Input: part model. Units: mm. Frame: model coordinates. Face numbers are marked on the shaded views. A direction names the side the tool comes from. Give positions to 0.01 mm unless a question says otherwise; leave off trailing zeros. Use a Markdown table: item, result. Add a question column.
1. Set-up query: the marked faces 1 and 2. Return all of +Z, -Z, +X, -X, +Y, -Y with unobstructed straight access to the full face (end or side cutting, diameter ignored); none if empty.
2. Material intervals for probe 1 along Y at (x, z) = (38.5, -221); probe 2 along Y at (x, z) = (11, 123.5); probe 3 along X at (y, z) = (5, 12), sorted ascending.
3. Pin query (flat end, axial travel): pin 1 (1.5 mm diameter, centred on x = 34, y = -27, fed in from +Z); pin 2 (12 mm diameter, centred on y = 27.5, z = 160, fed in from -X); pin 3 (4 mm diameter, centred on x = 12.5, z = 217.5, fed in from -Y). Return the tip coordinate at first contact, or that it passes through.
```python
from build123d import *


with BuildPart() as f1:
    # F0 (on Front) → F1 (revolve)
    with BuildSketch(Plane.XZ):
        with BuildLine():
            Line((32.97646, -255.911327), (32.97646, 284.373549))
            Line((32.97646, 284.373549), (7.57646, 284.373549))
            Line((7.57646, 284.373549), (7.57646, 248.330043))
            add(Edge.make_bspline(
                [(7.57646, 127), (7.57646, 169.495269), (7.57646, 210.378019), (7.57646, 248.330043)],
                knots=[0, 0, 0, 0, 121.330043, 121.330043, 121.330043, 121.330043], degree=3))
            add(Edge.make_bspline(
                [(7.57646, 0), (7.57646, 43.884717), (7.57646, 89.199349), (7.57646, 127)],
                knots=[0, 0, 0, 0, 127, 127, 127, 127], degree=3))
            add(Edge.make_bspline(
                [(6.467091, -127), (20.825056, -92.807998), (7.57646, -20.899639), (7.57646, 0)],
                knots=[0, 0, 0, 0, 127.004845, 127.004845, 127.004845, 127.004845], degree=3))
            add(Edge.make_bspline(
                [(6.467091, -254), (21.641339, -234.98531), (-10.096919, -166.445472), (6.467091, -127)],
                knots=[0, 0, 0, 0, 127, 127, 127, 127], degree=3))
            ThreePointArc((6.467091, -254), (4.699815, -255.408622), (2.49646, -255.911327))
            Line((2.49646, -255.911327), (-0.04354, -255.911327))
            ThreePointArc((-0.04354, -255.911327), (-3.635642, -257.399224), (-5.12354, -260.991327))
            Line((-5.12354, -260.991327), (-5.12354, -268.611327))
            Line((-5.12354, -268.611327), (32.97646, -268.611327))
            Line((32.97646, -268.611327), (32.97646, -255.911327))
        make_face()
    revolve(axis=Axis((32.97646, 0, 14.231111), (0, 0, -1)))


solid = f1.part
```
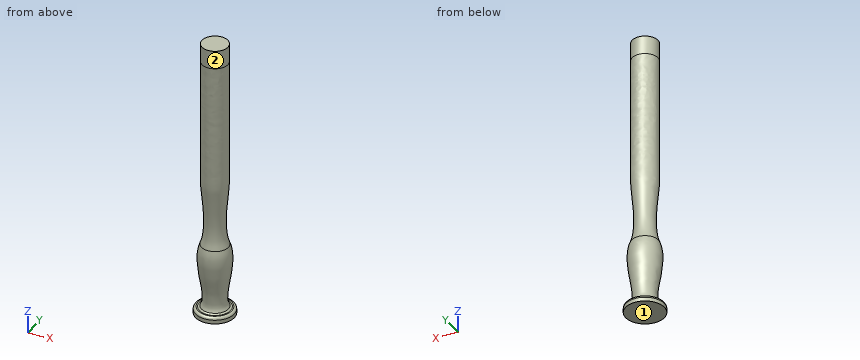
Result sheet:
| question | item | result |
|---|---|---|
| 1 | face 1 | -Z, +X, -X, +Y, -Y |
| 1 | face 2 | +Z |
| 2 | probe 1 | y = -22.84 to 22.84 |
| 2 | probe 2 | y = -12.74 to 12.74 |
| 2 | probe 3 | x = 8.07 to 57.88 |
| 3 | pin 1 | stops at z = -126.42 |
| 3 | pin 2 | stops at x = 19.45 |
| 3 | pin 3 | stops at y = -17.43 |
